Geometry: final body of the model. Coordinates: model frame, mm. A direction names the side the tool comes from. Give positions to 0.01 mm unless a question says otherwise; leave off trailing zeros. Write each loop counter-clockwise with the first axis right and the second up, starting at its lowest first coordinate (ties: lowest second). Pieces come first, ordered by that corner, then holes. Notation, with made-up numbers: M 53.5,-11 L 70.5,-11 A29 ccw 70.5,23 Z; hole C 51.5,4.5 d6. An arc over 180 degrees is marked long. Answer as a JSON object with one key per item and string values.
from build123d import *

# Parameters (mm, degrees)
SKETCH2_W           = 55
SKETCH2_H           = 6
BOSS_EXTRUDE8_DEPTH = 2
SKETCH4_R           = 0.3
CUT_EXTRUDE3_DEPTH  = 2
CUT_EXTRUDE4_START  = -2
SKETCH5_R           = 0.3
CUT_EXTRUDE4_DEPTH  = 2


with BuildPart() as part:
    # Sketch2 → Boss-Extrude8 (new body)
    with BuildSketch(Plane.XY):
        with Locations((0, -3)):
            Rectangle(SKETCH2_W, SKETCH2_H)
        with BuildLine():
            ThreePointArc((-27.5, -6), (-30.328427125, -7.171572875), (-31.5, -10))
            Line((-31.5, -10), (-31.5, -12))
            Line((-31.5, -12), (-33.5, -12))
            Line((-33.5, -12), (-33.5, -6))
            ThreePointArc((-33.5, -6), (-31.742640687, -1.757359313), (-27.5, 0))
            Line((-27.5, 0), (-27.5, -6))
        make_face()
        with BuildLine():
            Line((27.5, -6), (27.5, 0))
            ThreePointArc((27.5, 0), (31.742640687, -1.757359313), (33.5, -6))
            Line((33.5, -6), (33.5, -12))
            Line((33.5, -12), (31.5, -12))
            Line((31.5, -12), (31.5, -10))
            ThreePointArc((31.5, -10), (30.328427125, -7.171572875), (27.5, -6))
        make_face()
    extrude(amount=BOSS_EXTRUDE8_DEPTH)

    # Sketch4 → Cut-Extrude3 (cut)
    with BuildSketch(Plane(origin=(33.5, 0, 0), x_dir=(0, 0, -1), z_dir=(1, 0, 0))):
        with Locations((-1, -11)):
            Circle(SKETCH4_R)
    extrude(amount=-CUT_EXTRUDE3_DEPTH, mode=Mode.SUBTRACT)

    # Sketch5 → Cut-Extrude4 (cut)
    with BuildSketch(Plane.ZY.offset(33.5).offset(CUT_EXTRUDE4_START)):
        with Locations(Location((1, -11, 0), (0, 0, 180))):
            Circle(SKETCH5_R)
    extrude(amount=CUT_EXTRUDE4_DEPTH, mode=Mode.SUBTRACT)


solid = part.part
1) Contact query for a flat-ended pin moving along its axis: P1, Ø1, axis at x = -8.5, y = -6, coming from the -Z side. Output: stop coordinate, or through.
Geometry check:
{"P1": "stops at z = 0"}
2) Line query: line 1 (X direction, y = -9.75, z = 1.2); line 2 (Y direction, x = -12, z = 1.85); line 3 (Z direction, x = -32.2, y = -11). Output: solid intervals per line, ascending. Write a range as from..to.
Geometry check:
{"line 1": "x = -33.5..-31.49, 31.49..33.5", "line 2": "y = -6..0", "line 3": "z = 0..0.7, 1.3..2"}
3) Pull-direction query (X, two-part tool) for faces 1 (the flat face through (33.5, -9, 1)), 2 (the cylindrical face through (-31.789, -1.804, 0.986)), 3 (the cylindrical face through (-30.297, -7.141, 0.986)), 4 (the cylindrical face through (30.359, -7.203, 0.986)); classes: pulls with the +X half, pulls with the -X half, needs draft (parallel to the pull), parting line crosses it, or undercut.
Geometry check:
{"face 1": "pulls with the +X half", "face 2": "pulls with the -X half", "face 3": "undercut", "face 4": "undercut"}
4) Set-up query: faces 5 (the flat face through (0, -6, 1)), 6 (the flat face through (0, 0, 1)). Return all of +Z, -Z, +X, -X, +Y, -Y with unobstructed straight access to the full face (end or side cutting, diameter ignored); none if empty.
Geometry check:
{"face 5": "+Z, -Z, -Y", "face 6": "+Z, -Z, +X, -X, +Y"}
5) Cut plane B-B on x = 22. Return loops of the section in (y, z).
Geometry check:
{"outline": "M -6,0 L 0,0 L 0,2 L -6,2 Z"}
6) Cut plane A-A on z = 1. Return loops of the section in (x, y), and give its area (3 significant figures).
Geometry check:
{"outline": "M -33.5,-12 L -31.5,-12 L -31.5,-11.3 L -33.5,-11.3 Z; M -33.5,-10.7 L -31.5,-10.7 L -31.5,-10 A4 cw -27.5,-6 L 27.5,-6 A4 cw 31.5,-10 L 31.5,-10.7 L 33.5,-10.7 L 33.5,-6 A6 ccw 27.5,0 L -27.5,0 A6 ccw -33.5,-6 Z; M 31.5,-12 L 33.5,-12 L 33.5,-11.3 L 31.5,-11.3 Z", "area": "415 mm2"}
7) Cut plane C-C on y = -1.5. Return loops of the section in (x, z).
Geometry check:
{"outline": "M -31.47,0 L 31.47,0 L 31.47,2 L -31.47,2 Z"}
